For this review, take the finished solid that the model builds, in its own axes (mm). A direction names the side the tool comes from. Round coordinates to 2 decimals unless told otherwise and drop trailing zeros. Write each loop counter-clockwise with the first axis right and the second up, starting at its lowest first coordinate (ties: lowest second). Pieces come first, ordered by that corner, then holes. Notation, with made-up numbers: (-33.75, 58) -> (5.25, 58) arc R14 cw to (5.25, 82) -> close; hole circle Ø8 at (51, -33.5). An arc over 180 degrees is marked (long way). Answer as CSV lines item,"result". Start each with the question number.
Item 1: Machinability: for faces 5 (the cylindrical face through (8.78, 3.96, 1.25)), 6 (the flat face through (-10, -18, 2.54)), which of the approach directions +Z, -Z, +X, -X, +Y, -Y give a long, thin tool a straight path to every point of the face, cutting with its end or side? Answer none if there is none.
Item 2: Mouldability with a two-part tool opening along Y and no side actions: class faces 1 (the cylindrical face through (-31.307, -3.864, 1.252)), 2 (the flat face through (-1, -25.4, 3)), 3 (the flat face through (1, -23.812, 4)), 4 (the flat face through (0, -24, 5.08)) as +Y half, -Y half, draft (parallel to the pull), parting line (faces both ways), or undercut.
Item 3: Take a section at A-A on x = -10.16. Give the boundary of the cut face in (y, z).
Item 4: Take a section at B-B on y = 10.16. Count the separate pieces of the cut face and the enclosed holes in it, then the cut area to 3 significant figures.
Item 5: For pin 1 Ø16.5 at (x, y) = (-30.48, -10.16) entering from +Z; pin 2 Ø10.5 at (x, y) = (35.5, 8) entering from +Z; pin 3 Ø23.5 at (x, y) = (36, -14) entering from +Z, all flat-tipped, find the tip position at first contact; note any pin that passes through.
Item 6: Wall thickness on probe 1 along X at (y, z) = (-20.5, 2.85); probe 2 along Y at (x, z) = (-10.16, 1.55); probe 3 along Y at (x, z) = (34, 3.6): over which ranges is each line inside the solid? List them lowest first. Write a range as from..to.
```python
from build123d import *

# Parameters (mm, degrees)
F1_DEPTH = 5.08
F0_W     = 5.08
F0_H     = 21.3788050804
F0_H_2   = 4.8673898391
F0_W_2   = 26.406345436
F0_W_3   = 15.186154564
F0_W_4   = 15.3763087159
F0_W_5   = 26.2161912841
F2_DEPTH = 3.81
F0_R     = 6.35
F3_DEPTH = 2.54


with BuildPart() as f1:
    # F0 (on Top) → F1 (new body)
    with BuildSketch(Plane.XY):
        with BuildLine():
            ThreePointArc((-50.8, -20.32), (-49.3121024484, -23.9121024484), (-45.72, -25.4))
            Line((-45.72, -25.4), (45.72, -25.4))
            ThreePointArc((45.72, -25.4), (49.3121024484, -23.9121024484), (50.8, -20.32))
            Line((50.8, -20.32), (50.8, 20.32))
            ThreePointArc((50.8, 20.32), (49.3121024484, 23.9121024484), (45.72, 25.4))
            Line((45.72, 25.4), (-45.72, 25.4))
            ThreePointArc((-45.72, 25.4), (-49.3121024484, 23.9121024484), (-50.8, 20.32))
            Line((-50.8, 20.32), (-50.8, -20.32))
        make_face()
        with BuildLine():
            ThreePointArc((-49.2125, 20.32), (-48.1895704333, 22.7895704333), (-45.72, 23.8125))
            Line((-45.72, 23.8125), (-22.806154564, 23.8125))
            Line((-22.806154564, 23.8125), (-17.726154564, 23.8125))
            Line((-17.726154564, 23.8125), (-2.54, 23.8125))
            Line((-2.54, 23.8125), (2.54, 23.8125))
            Line((2.54, 23.8125), (17.9163087159, 23.8125))
            Line((17.9163087159, 23.8125), (22.9963087159, 23.8125))
            Line((22.9963087159, 23.8125), (45.72, 23.8125))
            ThreePointArc((45.72, 23.8125), (48.1895704333, 22.7895704333), (49.2125, 20.32))
            Line((49.2125, 20.32), (49.2125, 2.4336949196))
            Line((49.2125, 2.4336949196), (49.2125, -2.4336949196))
            Line((49.2125, -2.4336949196), (49.2125, -20.32))
            ThreePointArc((49.2125, -20.32), (48.1895704333, -22.7895704333), (45.72, -23.8125))
            Line((45.72, -23.8125), (22.9963087159, -23.8125))
            Line((22.9963087159, -23.8125), (17.9163087159, -23.8125))
            Line((17.9163087159, -23.8125), (2.54, -23.8125))
            Line((2.54, -23.8125), (-2.54, -23.8125))
            Line((-2.54, -23.8125), (-17.726154564, -23.8125))
            Line((-17.726154564, -23.8125), (-22.806154564, -23.8125))
            Line((-22.806154564, -23.8125), (-45.72, -23.8125))
            ThreePointArc((-45.72, -23.8125), (-48.1895704333, -22.7895704333), (-49.2125, -20.32))
            Line((-49.2125, -20.32), (-49.2125, -2.4336949196))
            Line((-49.2125, -2.4336949196), (-49.2125, 2.4336949196))
            Line((-49.2125, 2.4336949196), (-49.2125, 20.32))
        make_face(mode=Mode.SUBTRACT)
    extrude(amount=F1_DEPTH)

    # F0 (on Top) → F2 (join)
    with BuildSketch(Plane.XY):
        with Locations((-20.266154564, 13.1230974598)):
            Rectangle(F0_W, F0_H)
        with Locations((-20.266154564, 0)):
            Rectangle(F0_W, F0_H_2)
        with Locations((-36.009327282, 0)):
            Rectangle(F0_W_2, F0_H_2)
        with Locations((-20.266154564, -13.1230974598)):
            Rectangle(F0_W, F0_H)
        with Locations((-10.133077282, 0)):
            Rectangle(F0_W_3, F0_H_2)
        with Locations((0, 13.1230974598)):
            Rectangle(F0_W, F0_H)
        with Locations((0, -13.1230974598)):
            Rectangle(F0_W, F0_H)
        Rectangle(F0_W, F0_H_2)
        with Locations((10.228154358, 0)):
            Rectangle(F0_W_4, F0_H_2)
        with Locations((20.4563087159, 0)):
            Rectangle(F0_W, F0_H_2)
        with Locations((20.4563087159, 13.1230974598)):
            Rectangle(F0_W, F0_H)
        with Locations((20.4563087159, -13.1230974598)):
            Rectangle(F0_W, F0_H)
        with Locations((36.104404358, 0)):
            Rectangle(F0_W_5, F0_H_2)
    extrude(amount=F2_DEPTH)

    # F0 (on Top) → F3 (join)
    with BuildSketch(Plane.XY):
        with BuildLine():
            Line((-22.806154564, 23.8125), (-45.72, 23.8125))
            ThreePointArc((-45.72, 23.8125), (-48.1895704333, 22.7895704333), (-49.2125, 20.32))
            Line((-49.2125, 20.32), (-49.2125, 2.4336949196))
            Line((-49.2125, 2.4336949196), (-22.806154564, 2.4336949196))
            Line((-22.806154564, 2.4336949196), (-22.806154564, 23.8125))
        make_face()
        with Locations((-30.48, 10.16)):
            Circle(F0_R, mode=Mode.SUBTRACT)
        with Locations((-10.133077282, 13.1230974598)):
            Rectangle(F0_W_3, F0_H)
        with Locations((-10.16, 10.16)):
            Circle(F0_R, mode=Mode.SUBTRACT)
        with Locations((10.228154358, 13.1230974598)):
            Rectangle(F0_W_4, F0_H)
        with Locations((10.16, 10.16)):
            Circle(F0_R, mode=Mode.SUBTRACT)
        with BuildLine():
            Line((45.72, 23.8125), (22.9963087159, 23.8125))
            Line((22.9963087159, 23.8125), (22.9963087159, 2.4336949196))
            Line((22.9963087159, 2.4336949196), (49.2125, 2.4336949196))
            Line((49.2125, 2.4336949196), (49.2125, 20.32))
            ThreePointArc((49.2125, 20.32), (48.1895704333, 22.7895704333), (45.72, 23.8125))
        make_face()
        with Locations((30.48, 10.16)):
            Circle(F0_R, mode=Mode.SUBTRACT)
        with BuildLine():
            Line((49.2125, -2.4336949196), (22.9963087159, -2.4336949196))
            Line((22.9963087159, -2.4336949196), (22.9963087159, -23.8125))
            Line((22.9963087159, -23.8125), (45.72, -23.8125))
            ThreePointArc((45.72, -23.8125), (48.1895704333, -22.7895704333), (49.2125, -20.32))
            Line((49.2125, -20.32), (49.2125, -2.4336949196))
        make_face()
        with Locations((30.48, -10.179114528)):
            Circle(F0_R, mode=Mode.SUBTRACT)
        with Locations((10.228154358, -13.1230974598)):
            Rectangle(F0_W_4, F0_H)
        with Locations((10.16, -10.16)):
            Circle(F0_R, mode=Mode.SUBTRACT)
        with Locations((-10.133077282, -13.1230974598)):
            Rectangle(F0_W_3, F0_H)
        with Locations((-10.16, -10.16)):
            Circle(F0_R, mode=Mode.SUBTRACT)
        with BuildLine():
            Line((-22.806154564, -2.4336949196), (-49.2125, -2.4336949196))
            Line((-49.2125, -2.4336949196), (-49.2125, -20.32))
            ThreePointArc((-49.2125, -20.32), (-48.1895704333, -22.7895704333), (-45.72, -23.8125))
            Line((-45.72, -23.8125), (-22.806154564, -23.8125))
            Line((-22.806154564, -23.8125), (-22.806154564, -2.4336949196))
        make_face()
        with Locations((-30.48, -10.16)):
            Circle(F0_R, mode=Mode.SUBTRACT)
    extrude(amount=F3_DEPTH)


solid = f1.part
```
Output values:
1,face 5,"+Z, -Z"
1,face 6,"+Z"
2,face 1,"undercut"
2,face 2,"-Y half"
2,face 3,"undercut"
2,face 4,"draft"
3,outline,"(-25.4, 0) -> (-16.51, 0) -> (-16.51, 2.54) -> (-23.81, 2.54) -> (-23.81, 5.08) -> (-25.4, 5.08) -> close; (-3.81, 0) -> (3.81, 0) -> (3.81, 2.54) -> (2.43, 2.54) -> (2.43, 3.81) -> (-2.43, 3.81) -> (-2.43, 2.54) -> (-3.81, 2.54) -> close; (16.51, 0) -> (25.4, 0) -> (25.4, 5.08) -> (23.81, 5.08) -> (23.81, 2.54) -> (16.51, 2.54) -> close"
4,separate pieces,"5"
4,enclosed holes,"0"
4,area,"156 mm^2"
5,pin 1,"stops at z = 3.81"
5,pin 2,"stops at z = 2.54"
5,pin 3,"stops at z = 5.08"
6,probe 1,"x = -50.8..-49.21, -22.81..-17.73, -2.54..2.54, 17.92..23, 49.21..50.8"
6,probe 2,"y = -25.4..-16.51, -3.81..3.81, 16.51..25.4"
6,probe 3,"y = -25.4..-23.81, -2.43..2.43, 23.81..25.4"
